Autodesk Inventor part; units mm, degrees
ref_plane "YZ Plane" through (0, 0, 0) normal (1, 0, 0) x (0, 1, 0)
ref_plane "XZ Plane" through (0, 0, 0) normal (0, 1, 0) x (-1, 0, 0)
ref_plane "XY Plane" through (0, 0, 0) normal (0, 0, 1) x (1, 0, 0)
sketch "スケッチ2" plane through (0, 0, 0) normal (0, 1, 0) x (-1, 0, 0)
  line L0 (-32.5, -11.25) -> (32.5, -11.25)
  line L1 (32.5, -11.25) -> (32.5, 11.25)
  line L2 (32.5, 11.25) -> (-32.5, 11.25)
  line L3 (-32.5, 11.25) -> (-32.5, -11.25)
  line L4 (-32.5, -11.25) -> (32.5, 11.25) construction
  line L5 (32.5, -11.25) -> (-32.5, 11.25) construction
  line L6 (-30, -8.75) -> (30, -8.75)
  line L7 (30, -8.75) -> (30, 8.75)
  line L8 (30, 8.75) -> (-30, 8.75)
  line L9 (-30, 8.75) -> (-30, -8.75)
  line L10 (-30, -8.75) -> (30, 8.75) construction
  line L11 (30, -8.75) -> (-30, 8.75) construction
  circle A0 centre (30, 8.75) radius 2.5
  circle A1 centre (30, -8.75) radius 2.5
  circle A2 centre (-30, 8.75) radius 2.5
  circle A3 centre (-30, -8.75) radius 2.5
  line L12 (-115, -18.25) -> (115, -18.25)
  line L13 (115, -18.25) -> (115, 18.25)
  line L14 (115, 18.25) -> (-115, 18.25)
  line L15 (-115, 18.25) -> (-115, -18.25)
  line L16 (-115, -18.25) -> (115, 18.25) construction
  line L17 (115, -18.25) -> (-115, 18.25) construction
  line L18 (-95, -18.25) -> (95, -18.25)
  line L19 (95, -18.25) -> (95, 18.25)
  line L20 (95, 18.25) -> (-95, 18.25)
  line L21 (-95, 18.25) -> (-95, -18.25)
  line L22 (-95, -18.25) -> (95, 18.25) construction
  line L23 (95, -18.25) -> (-95, 18.25) construction
  point P0 (0, 0)
  dimension "d10" = 65
  dimension "d11" = 22.5
  dimension "d12" = 60
  dimension "d13" = 17.5
  dimension "d14" = 230
  dimension "d15" = 36.5
  dimension "d16" = 190
sketch "スケッチ4" plane through (0, 0, 0) normal (1, 0, 0) x (0, 1, 0)
  point P0 (0, 0)
sketch "スケッチ5" plane through (0, 0, 0) normal (1, 0, 0) x (0, 1, 0)
  circle A0 centre (0, 0) radius 18.25
  line L0 (0, 0) -> (0, 6)
  line L1 (0, 6) -> (0, -6)
  circle A1 centre (0, 6) radius 3
  circle A2 centre (0, -6) radius 9
  circle A3 centre (0, 6) radius 9
  circle A4 centre (0, -6) radius 3
  line L2 (0, 6) -> (5.2915, 0)
  circle A5 centre (5.2915, 0) radius 5
  circle A6 centre (5.2915, 0) radius 4.5
  circle A7 centre (5.2915, 0) radius 5.5
  line L3 (0, 0) -> (0, 11.25)
  line L4 (0, 11.25) -> (0, -11.25)
  line L5 (5.2915, 5.5) -> (5.2915, -5.5)
  line L6 (0, 11.25) -> (-1.2, 11.25)
  line L7 (-1.2, 11.25) -> (-1.2, -11.25)
  line L8 (-1.2, -11.25) -> (0, -11.25)
  line L9 (-1.2, 11.25) -> (-9.2, 11.25)
  line L10 (-1.2, -11.25) -> (-9.2, -11.25)
  line L11 (-9.2, -11.25) -> (-9.2, 11.25)
  line L12 (-9.2, 11.25) -> (-10.4, 11.25)
  line L13 (-10.4, 11.25) -> (-10.4, -11.25)
  line L14 (-10.4, -11.25) -> (-9.2, -11.25)
  circle A8 centre (0, 0) radius 16
  line L15 (0, 11.25) -> (1.5, 11.25)
  line L16 (1.5, 11.25) -> (1.5, -11.25)
  line L17 (1.5, -11.25) -> (0, -11.25)
  line L18 (5.2915, 5.5) -> (1.5, 5.5)
  line L19 (5.2915, -5.5) -> (1.5, -5.5)
  circle A9 centre (5.2915, 0) radius 6.6802
  point P0 (0, 1.5)
  point P1 (0, -1.5)
  point P2 (1.5, -3.9843)
  point P3 (1.5, 3.9843)
  dimension "d28" = 36.5
  dimension "d29" = 6
  dimension "d30" = 12
  dimension "d31" = 6
  dimension "d32" = 18
  dimension "d33" = 8
  dimension "d34" = 9
  dimension "d35" = 11
  dimension "d36" = 11.25
  dimension "d37" = 22.5
  dimension "d39" = 1.2
  dimension "d40" = 8
  dimension "d41" = 1.2
  dimension "d42" = 32
  dimension "d43" = 1.5
ref_plane "作業平面1" through (16.5, 5.2915, 0) normal (1, 0, 0) x (0, 0, 1)
sketch "スケッチ6" plane through (16.5, 5.2915, 0) normal (1, 0, 0) x (0, 0, 1)
  line L0 (0, 5.2915) -> (6, 5.2915)
  line L1 (-11.25, 5.2915) -> (11.25, 5.2915)
  line L2 (6, 5.2915) -> (-6, 5.2915)
  circle A0 centre (6, 5.2915) radius 1.05
  circle A1 centre (-6, 5.2915) radius 1.05
  circle A2 centre (0, 5.2915) radius 16
  circle A3 centre (0, 0) radius 5
  line L3 (0, 0) -> (0, 3)
  line L4 (0, 3) -> (0, -5.5)
  arc A4 (-5.5, 0) -> (5.5, 0) centre (0, 0) ccw
  line L5 (0, 3) -> (1, 3)
  line L6 (1, 3) -> (-1, 3)
  line L7 (-1, 3) -> (-1, -5.4083)
  line L8 (1, 3) -> (1, -5.4083)
  circle A5 centre (6, 5.2915) radius 9
  circle A6 centre (-6, 5.2915) radius 9
  line L9 (0, 5.2915) -> (0, -2.7085)
  circle A7 centre (0, -2.7085) radius 8
  circle A8 centre (6, 5.2915) radius 10
  circle A9 centre (-6, 5.2915) radius 10
  line L10 (0, 5.2915) -> (0, -5.7085)
  line L11 (0, -5.7085) -> (-11.619, -5.7085)
  line L12 (0, -5.7085) -> (11.619, -5.7085)
  line L13 (0, -5.7085) -> (9.5, -5.7085)
  line L14 (9.5, -5.7085) -> (-9.5, -5.7085)
  circle A10 centre (0, 5.2915) radius 18
  line L15 (1, -5.4083) -> (1, -8.2085)
  line L16 (-1, -5.4083) -> (-1, -8.2085)
  line L17 (0, 5.2915) -> (0, 6.4915)
  line L18 (0, 6.4915) -> (0, 14.4915)
  line L19 (0, 14.4915) -> (0, 15.6915)
  line L20 (0, 15.6915) -> (-11.25, 15.6915)
  line L21 (-11.25, 15.6915) -> (11.25, 15.6915)
  line L22 (11.25, 15.6915) -> (11.25, 14.4915)
  line L23 (11.25, 14.4915) -> (0, 14.4915)
  line L24 (-11.25, 14.4915) -> (-11.25, 15.6915)
  line L25 (0, 14.4915) -> (-11.25, 14.4915)
  line L26 (0, 15.6915) -> (8.75, 15.6915)
  line L27 (8.75, 15.6915) -> (-8.75, 15.6915)
  line L28 (11.25, 15.6915) -> (11.25, 17.1915)
  line L29 (11.25, 17.1915) -> (-11.25, 17.1915)
  line L30 (-11.25, 17.1915) -> (-11.25, 15.6915)
  line L31 (6, 17.1915) -> (6, 18.6915)
  line L32 (-6, 17.1915) -> (-6, 18.6915)
  circle A11 centre (6, 18.6915) radius 2.5
  circle A12 centre (-6, 18.6915) radius 2.5
  line L33 (6, 21.1915) -> (-6, 21.1915)
  line L34 (9.5, -5.7085) -> (12, -5.7085)
  line L35 (-9.5, -5.7085) -> (-12, -5.7085)
  line L36 (6, 18.6915) -> (8.5, 18.6915)
  line L37 (-6, 18.6915) -> (-8.5, 18.6915)
  circle A13 centre (0, 0) radius 4.5
  circle A14 centre (-6, 5.2915) radius 1.5
  circle A15 centre (6, 5.2915) radius 1.5
  circle A16 centre (6, 18.6915) radius 1.65
  circle A17 centre (-6, 18.6915) radius 1.65
  line L38 (9.5, -5.7085) -> (9.5, -6.2085)
  line L39 (9.5, -6.2085) -> (-9.5, -6.2085)
  line L40 (-9.5, -6.2085) -> (-9.5, -5.7085)
  circle A18 centre (-9.5, -6.2085) radius 1.65
  circle A19 centre (9.5, -6.2085) radius 1.65
  circle A20 centre (9.5, -6.2085) radius 2.5
  circle A21 centre (-9.5, -6.2085) radius 2.5
  line L41 (-12, -6.2085) -> (-8.5, 18.6915)
  line L42 (12, -6.2085) -> (8.5, 18.6915)
  line L43 (9.5, -8.7085) -> (-9.5, -8.7085)
  line L44 (1, -8.7085) -> (1, -8.0358)
  line L45 (-1, -8.7085) -> (-1, -8.2085)
  point P0 (1, -4.3875)
  point P1 (-1, -4.3875)
  point P2 (-4.4567, 20.6583)
  point P3 (-8.495, 18.8501)
  point P4 (4.4567, 20.6583)
  point P5 (8.495, 18.8501)
  point P6 (1.7861, 21.1915)
  point P7 (-1.7861, 21.1915)
  point P8 (11.9031, -5.5193)
  point P9 (11.8759, -5.4306)
  point P10 (11.8887, -5.4164)
  dimension "d54" = 6
  dimension "d55" = 12
  dimension "d56" = 2.1
  dimension "d57" = 2.1
  dimension "d58" = 32
  dimension "d59" = 10
  dimension "d60" = 3
  dimension "d61" = 1
  dimension "d62" = 2
  dimension "d65" = 18
  dimension "d66" = 18
  dimension "d67" = 8
  dimension "d68" = 11
  dimension "d69" = 9.5
  dimension "d70" = 19
  dimension "d73" = 36
  dimension "d76" = 1.2
  dimension "d77" = 8
  dimension "d78" = 1.2
  dimension "d79" = 8.75
  dimension "d80" = 17.5
  dimension "d81" = 1.5
  dimension "d82" = 1.5
  dimension "d83" = 5
  dimension "d84" = 5
  dimension "d97" = 3
  dimension "d98" = 3
  dimension "d109" = 3.3
  dimension "d110" = 3.3
  dimension "d111" = 0.5
  dimension "d112" = 3.3
  dimension "d113" = 3.3
  dimension "d114" = 5
  dimension "d115" = 5
extrude "押し出し11" add sketch "スケッチ6" against normal blind 4 contours L17 L18 A6 L0 | A7 A5 L1 | A7 A6 A3 L9 | L0 A6 A7 | L9 A3 A5 A7 | L1 A5 L18 L17 | A6 A5 A9 L0 | L0 A9 A7 A6 | A5 A7 A8 L1 | L1 A8 A6 A5 | L9 A13 A5 A3 | A3 A6 A13 L9 | A7 A9 A3 A6 | A5 A3 A8 A7 | A9 A5 L42 L1 A15 L0 | L0 A15 L1 L42 A5 A7 A9 | L18 A9 A5 | A6 A8 L18 | A8 A7 A6 L41 L1 A14 | L1 A14 L41 A6 A8 | A3 A9 A13 A6 | A5 A13 A8 A3 | A13 A6 L8 L5 L9 | L9 L6 L7 A5 A13 | A7 A5 A3 A9 | A8 A3 A6 A7 | A15 L1 A0 L0 | L0 A0 L1 A15 | A9 A8 L23 L42 A5 | A6 L41 L25 A9 A8 | L18 L23 A8 | A9 L25 L18 | A14 L1 A1 | L1 A1 A14 | A3 A5 A13 A9 | A13 A9 L8 A6 | A8 A13 A6 A3 | A5 L7 A8 A13 | L5 L8 A6 L4 L3 | L3 L4 A5 L7 L6 | A7 A21 A9 L41 A6 | A6 A4 A9 A21 A7 | A0 L1 L0 | L0 L1 A0 | L23 L19 L21 L42 A8 | A8 L42 L23 | L25 L41 A9 | A9 L41 L20 L19 L25 | A1 L1 | L1 A1 | A13 A5 L8 A9 | L8 A9 A5 A6 | A6 A13 A9 A3 | A3 A9 A4 A6 | A8 L7 A6 A13 | A5 A6 A8 L7 | A7 A20 A8 A4 A5 | A5 L42 A8 A20 A7 | A21 A9 A7 | A7 A9 A21 | L20 L41 L29 A12 A11 L42 L21 | A5 A4 A8 A3 | A3 A8 A13 A5 | L8 A5 A9 | A5 A9 L4 | L4 A8 A6 | A9 A13 L7 A3 | A3 L7 A4 A9 | A6 L7 A9 A13 | A8 A6 L7 | A20 A8 A7 | A7 A8 A20 | A9 A21 A2 L41 | A4 L16 L11 A21 A9 | A9 A21 L11 A7 | A7 L11 A18 A2 A21 A9 | A8 A4 L8 A3 | A3 L8 A13 A8 | A13 A8 L8 A5 | L8 A8 A9 A5 | A8 L8 A13 L4 | A9 L7 A6 A8 | L4 A13 L7 A9 | L7 A13 L4 A3 | A3 L4 A4 L7 | A9 L7 A13 | A8 A20 L12 L15 A4 | L42 A2 A20 A8 | A8 A20 A2 L12 A19 A7 | A7 L12 A20 A8 | A2 A21 L41 | A4 L10 L11 L16 | L11 A21 L39 A7 | A7 L39 A18 L11 | L11 L16 L39 A21 | A2 L35 L41 A21 | L29 A11 L42 | L41 A12 L29 | L8 A4 L4 A3 | A3 L4 A13 L8 | A13 L8 A8 | L15 L12 L10 A4 | L12 A19 L39 A7 | A7 L39 A20 L12 | A20 L42 L34 A2 | A20 L39 L15 L12 | L11 L12 L15 L39 L16 | L39 A21 A7 | A7 A21 A2 A18 L39 | L39 L16 L45 L43 A7 A21 | L11 A18 A2 | A2 A18 A21 L41 L35 | A11 L29 A16 | L29 A16 L36 A11 | L36 A16 A2 A11 | A12 L37 A17 L29 | L29 A17 A12 | A12 A2 A17 L37 | L39 A19 A2 A20 A7 | A7 A20 L39 | L34 L42 A20 A2 A19 | A2 A19 L12 | A20 A7 L43 L44 L15 L39 | L39 L15 L44 L43 L45 L16 | A7 L43 A2 A21 | A2 A16 A11 | A11 A2 A16 L29 | L29 A12 A2 L33 A11 | L29 A17 A2 A12 | A12 A2 A17 | A20 A2 L43 A7 | A2 L43 A21 | A11 A2 L33 | L33 A2 A12 | A20 L43 A2 picked at (5.1751, 14.7127) picked at (-5.1751, 14.7127)
hole "穴2" at (16.5, 0, 0) direction (-1, 0, 0) diameter 3.3 end through all
properties part number "ikafly1c"
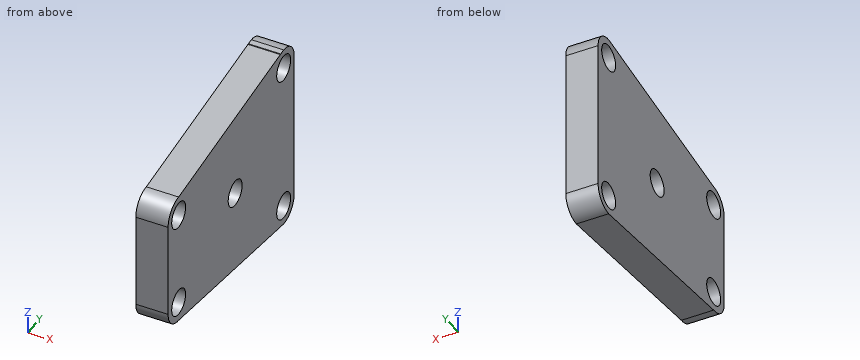
Here's how the part is built. I have some questions about the finished solid (model axes, mm). Coordinates: 2 decimals unless noted, no trailing zeros. Write each loop counter-clockwise with the first axis right and the second up, starting at its lowest first coordinate (ties: lowest second). Pieces come first, ordered by that corner, then holes.
Item 1: I want a section at A-A on z = 0. Write out the boundary of the cut face in (x, y).
Item 2: I want a section at B-B on x = 14.15. Count the separate pieces of the cut face and the enclosed holes in it, and give its area (3 significant figures).
Item 3: I want a section at C-C on y = 0. Write out the boundary of the cut face in (x, z).
Item 4: Will this pin go through, and if not, where does the flat tip stop? pin 1 (2 mm diameter, centred on x = 15.5, y = 9, fed in from -Z).
Item 5: If I drill on line 1 (Z direction, x = 14.6, y = -13.4); line 2 (Y direction, x = 15.2, z = 6); line 3 (Y direction, x = 13.75, z = 0), over which ranges is the centre line in solid material (lowest first)?
Item 6: I want a section at D-D on y = -12.5. Write out the boundary of the cut face in (x, z), and give its area (3 significant figures).
Findings below:
1. outline: (12.5, -15.9) - (16.5, -15.9) - (16.5, -1.65) - (12.5, -1.65) - close; (12.5, 1.65) - (16.5, 1.65) - (16.5, 14) - (12.5, 14) - close
2. separate pieces: 1
2. enclosed holes: 5
2. area: 565 mm2
3. outline: (12.5, -10.38) - (16.5, -10.38) - (16.5, -1.65) - (12.5, -1.65) - close; (12.5, 1.65) - (16.5, 1.65) - (16.5, 10.38) - (12.5, 10.38) - close
4. pin 1: stops at z = -11.79
5. line 1: z = -8.5 to -7.65, -4.35 to 4.35, 7.65 to 8.5
5. line 2: y = -15.9 to -15.05, -11.75 to 14
5. line 3: y = -15.9 to -1.65, 1.65 to 14
6. outline: (12.5, -8.63) - (16.5, -8.63) - (16.5, -7.38) - (12.5, -7.38) - close; (12.5, -4.62) - (16.5, -4.62) - (16.5, 4.62) - (12.5, 4.62) - close; (12.5, 7.38) - (16.5, 7.38) - (16.5, 8.63) - (12.5, 8.63) - close
6. area: 46.9 mm2
